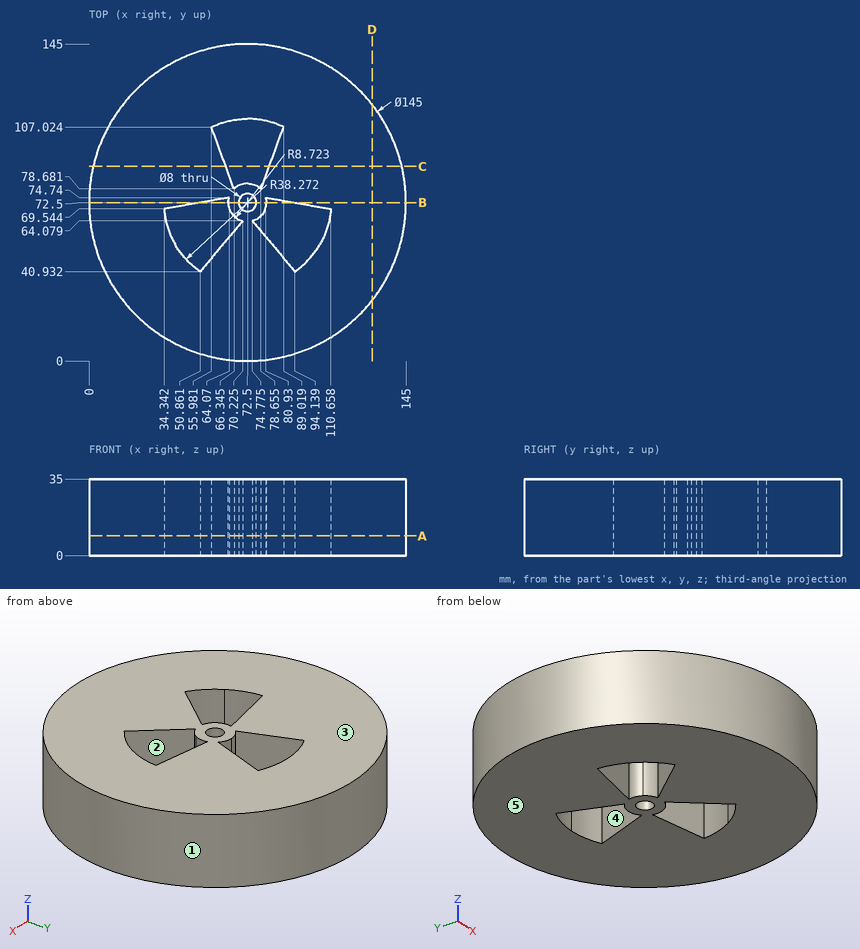
Design review of the part shown in the three views and the two pictorial views. Dimensions are in mm from the part's minimum x, y and z. A direction names the side the tool comes from. Round coordinates to 2 decimals unless told otherwise and drop trailing zeros. Loops run counter-clockwise (first coordinate to the right, second up) from the corner with the lowest first, then second, coordinate; pieces in that order, holes last. Notation, with made-up numbers: M -39.5,53.5 L 11.5,53.5 A5 ccw 11.5,60.5 Z; hole C 9,13 d3. An arc over 180 degrees is marked long. Answer as a JSON object with one key per item and string values.
Item 1: We need section B-B, the plane y = 72.5. State the section outline as (x, z) points, and give its area (3 significant figures).
Check sheet entries:
{"outline": "M 0,0 L 51.25,0 L 51.25,35 L 0,35 Z; M 63.78,0 L 68.5,0 L 68.5,35 L 63.78,35 Z; M 76.5,0 L 81.22,0 L 81.22,35 L 76.5,35 Z; M 93.75,0 L 145,0 L 145,35 L 93.75,35 Z", "area": "3,920 mm2"}
Item 2: Clearance check with flat-ended pins moving along their axes: P1, Ø2, axis at x = 27.5, z = 26, coming from the -Y side; P2, Ø1.5, axis at y = 71.5, z = 5.5, coming from the +X side; P3, Ø2, axis at x = 89, z = 12.5, coming from the -Y side; P4, Ø8, axis at x = 85, y = 59.5, coming from the +Z side. State where each tip first meets the part, or that it passes through.
Check sheet entries:
{"P1": "y = 14.88", "P2": "x = 145", "P3": "y = 1.68", "P4": "through"}
Item 3: The part is to be moulded in two halves that separate along X. For the marked faces 1, 2 and 3, say which applies: +X half, -X half, draft (parallel to the pull), parting line (faces both ways), or undercut.
Check sheet entries:
{"face 1": "parting line", "face 2": "undercut", "face 3": "draft"}
Item 4: For line 1 along Y through (x, z) = (72, 8); line 2 along X through (y, z) = (45.5, 27) (1 decimal); line 3 along Y through (x, z) = (77.5, 24) (1 decimal), list the stretches that pass through material, from the lowest coordinate up.
Check sheet entries:
{"line 1": "0 to 68.53, 76.47 to 81.21, 110.77 to 145", "line 2": "5.2 to 45.4, 54.7 to 90.3, 99.6 to 139.8", "line 3": "0.2 to 60.8, 65.4 to 79.6, 110.4 to 144.8"}
Item 5: We need section D-D, the plane x = 129.5. State the section outline as (y, z) points, and give its area (3 significant figures).
Check sheet entries:
{"outline": "M 27.7,0 L 117.3,0 L 117.3,35 L 27.7,35 Z", "area": "3,140 mm2"}
Item 6: We need section C-C, the plane y = 89. State the section outline as (x, z) points, and give its area (3 significant figures).
Check sheet entries:
{"outline": "M 1.9,0 L 62.57,0 L 62.57,35 L 1.9,35 Z; M 82.43,0 L 143.1,0 L 143.1,35 L 82.43,35 Z", "area": "4,250 mm2"}
Item 7: We need section A-A, the plane z = 9. State the section outline as (x, y) points (1 decimal), and give its area (3 significant figures).
Check sheet entries:
{"outline": "C 72.5,72.5 d145; hole M 34.3,69.5 A38.3 ccw 50.9,40.9 L 70.2,64.1 A8.7 cw 64.1,74.7 Z; hole M 56,107 L 66.3,78.7 A8.7 cw 78.7,78.7 L 89,107 A38.3 ccw Z; hole C 72.5,72.5 d8; hole M 74.8,64.1 L 94.1,40.9 A38.3 ccw 110.7,69.5 L 80.9,74.7 A8.7 cw Z", "area": "14,300 mm2"}
Item 8: Tool access review of the marked faces 4 and 5: name each direction out of +Z, -Z, +X, -X, +Y, -Y from which nothing blocks a thin tool from reaching the whole face with its end or side.
Check sheet entries:
{"face 4": "+Z, -Z", "face 5": "-Z, +X, -X, +Y, -Y"}
